```python
from build123d import *

# Parameters (mm, degrees)
F1_DEPTH = 3.81
F2_R     = 14.4183886526
F2_R_2   = 14.9688015553
F2_R_3   = 13.8673627738
F2_R_4   = 14.6123692091
F2_R_5   = 14.6887640566
F2_R_6   = 13.7656196585
F2_R_7   = 6.5271201163
F2_R_8   = 3.1776406916
F2_R_9   = 2.2295804693
F2_R_10  = 1.3934876863
F2_R_11  = 3.1159324266
F2_R_12  = 2.3730237654
F2_R_13  = 1.5391584656
F2_R_14  = 2.962596298
F2_R_15  = 2.2032977608
F2_R_16  = 2.9560338706
F2_R_17  = 2.3730243841
F2_R_18  = 1.4346833287
F2_R_19  = 1.5391578396
F2_R_20  = 2.8008757636
F2_R_21  = 2.094873282
F2_R_22  = 1.672185105
F2_R_23  = 3.2080502358
F2_R_24  = 2.1677587647
F2_R_25  = 1.3934881637
F3_DEPTH = 3.811
F4_SCALE = 0.6
F6_DEPTH = 2.287


with BuildPart() as f1:
    # F0 (on Top) → F1 (new body)
    with BuildSketch(Plane.XY):
        Polygon((21.5040096467, 37.2460372746), (-21.5040096467, 37.2460372746), (-43.0080192935, 0), (-21.5040096467, -37.2460372746), (21.5040096467, -37.2460372746), (43.0080192935, 0), align=None)
    extrude(amount=F1_DEPTH)

    # F2 (on face) → F3 (cut, through all)
    with BuildSketch(Plane.XY.offset(3.81)):
        with Locations((0, 37.2460372746)):
            Circle(F2_R)
        with Locations((-32.2560144701, 18.6230186373)):
            Circle(F2_R_2)
        with Locations((-32.2560144701, -18.6230186373)):
            Circle(F2_R_3)
        with Locations((0, -37.2460372746)):
            Circle(F2_R_4)
        with Locations((32.2560144701, -18.6230186373)):
            Circle(F2_R_5)
        with Locations((31.3001683758, 20.2785926369)):
            Circle(F2_R_6)
        Circle(F2_R_7)
        with Locations((-12.8094833344, 20.49517259)):
            Circle(F2_R_8)
        with Locations((-9.065172635, 13.0065521225)):
            Circle(F2_R_9)
        with Locations((-5.9120692313, 7.2915516794)):
            Circle(F2_R_10)
        with Locations((11.8241384625, 21.8746569008)):
            Circle(F2_R_11)
        with Locations((9.0651735663, 14.3860345706)):
            Circle(F2_R_12)
        with Locations((5.9120692313, 8.2768965513)):
            Circle(F2_R_13)
        with Locations((27.5896564126, 0)):
            Circle(F2_R_14)
        with Locations((18.9186222851, 0)):
            Circle(F2_R_15)
        with Locations((13.5977584869, -23.2541374862)):
            Circle(F2_R_16)
        with Locations((9.4593111426, -15.1743106544)):
            Circle(F2_R_17)
        with Locations((5.1237940788, -9.6563789994)):
            Circle(F2_R_18)
        with Locations((10.4446560144, 0)):
            Circle(F2_R_19)
        with Locations((-14.3860345706, -21.4805174619)):
            Circle(F2_R_20)
        with Locations((-10.4446560144, -14.7801730782)):
            Circle(F2_R_21)
        with Locations((-7.2915512137, -9.2622414231)):
            Circle(F2_R_22)
        with Locations((-26.2101721019, 0)):
            Circle(F2_R_23)
        with Locations((-17.9332755506, 0)):
            Circle(F2_R_24)
        with Locations((-11.2329311669, 0)):
            Circle(F2_R_25)
    extrude(amount=-F3_DEPTH, mode=Mode.SUBTRACT)


with BuildPart() as f1_1:
    # F4: moved
    add(f1.part.scale(F4_SCALE))

    # F5 (on face) → F6 (cut, through all)
    with BuildSketch(Plane.XY.offset(2.286)):
        Polygon((2.2348568425, 7.9494534601), (3.6136271371, 11.252985526), (0.8978448914, 13.585121549), (-2.1593711371, 11.7229288117), (-1.333052308, 8.2398943834), align=None)
        with BuildLine():
            ThreePointArc((-11.0931667862, 7.648402428), (-11.1968162546, 7.4148027366), (-11.3070701633, 7.1842466615))
            Line((-11.3070701633, 7.1842466615), (-11.2320397263, 3.9913941449))
            Line((-11.2320397263, 3.9913941449), (-7.8024840145, 2.9654900284))
            Line((-7.8024840145, 2.9654900284), (-5.7670002214, 5.9101695295))
            Line((-5.7670002214, 5.9101695295), (-7.9385577654, 8.7559856636))
            Line((-7.9385577654, 8.7559856636), (-11.0931667862, 7.648402428))
        make_face()
        Polygon((-6.4694317065, -5.274404355), (-8.0018570639, -2.0392839306), (-11.5521849025, -2.4969998625), (-12.2139828207, -6.0150042899), (-9.0726685891, -7.7315346668), align=None)
        Polygon((-2.2348568425, -7.9494534601), (-3.6136271371, -11.252985526), (-0.8978448914, -13.585121549), (2.1593711371, -11.7229288117), (1.333052308, -8.2398943834), align=None)
        with BuildLine():
            Line((5.7670002214, -5.9101695295), (7.9385577654, -8.7559856636))
            Line((7.9385577654, -8.7559856636), (11.3097934002, -7.5723448233))
            ThreePointArc((11.3097934002, -7.5723448233), (11.3128298264, -7.5655706667), (11.3158719575, -7.5587990702))
            Line((11.3158719575, -7.5587990702), (11.2320397263, -3.9913941449))
            Line((11.2320397263, -3.9913941449), (7.8024840145, -2.9654900284))
            Line((7.8024840145, -2.9654900284), (5.7670002214, -5.9101695295))
        make_face()
        Polygon((8.0018570639, 2.0392839306), (11.5521849025, 2.4969998625), (12.2139828207, 6.0150042899), (9.0726685891, 7.7315346668), (6.4694317065, 5.274404355), align=None)
    extrude(amount=-F6_DEPTH, mode=Mode.SUBTRACT)


solid = f1_1.part
```
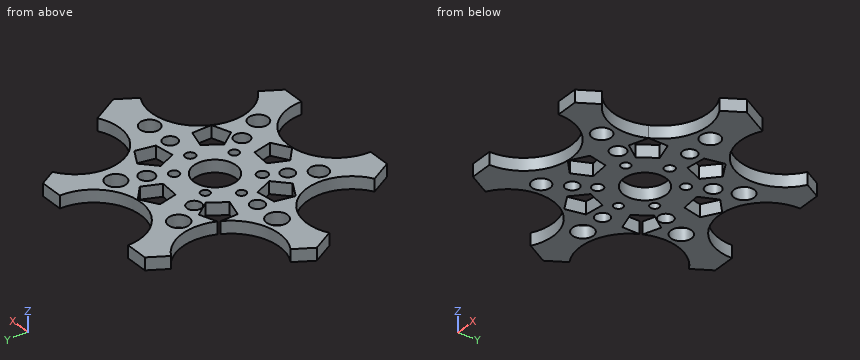
CAD build for the part. Positions are in the model's coordinates, mm. Round coordinates to 2 decimals unless told otherwise and drop trailing zeros. Order: outer loops, then holes, each group sorted by start corner. A loop starts at its lowest first (then second) coordinate and runs counter-clockwise, first axis right, second up. Notation, with made-up numbers: (-38, 67) -> (16, 67) arc R20 cw to (16, 92) -> close; hole circle Ø11 at (-39.5, 64). An arc over 180 degrees is marked (long way). One line per question, with ' | ' between items.
Q1. Slice it at C-C (z = 0.5). Give the number of separate pieces and of enclosed holes in the cut face, then the cut area to 3 significant figures.
Completed:
separate pieces: 1 | enclosed holes: 23 | area: 735 mm^2
Q2. Probe probe 1 along Y at (x, z) = (14, 0.25); probe 2 along X at (y, z) = (-7, 1.3); probe 3 along X at (y, z) = (-17, 1.65). List the from-to ranges inside material, lowest first.
Completed:
probe 1: y = -20.45 to -18.17, -4.17 to 5.43, 18.9 to 20.45 | probe 2: x = -12.16 to -10.41, -8.3 to 6.6, 11.3 to 11.59 | probe 3: x = -13.41 to -6.95, 6.95 to 12.74
Q3. Slice it at B-B (x = 0). Write the cut outline in (y, z).
Completed:
outline: (-13.58, 0) -> (-13.04, 0) -> (-13.04, 2.29) -> (-13.58, 2.29) -> close; (-8.13, 0) -> (-3.92, 0) -> (-3.92, 2.29) -> (-8.13, 2.29) -> close; (3.92, 0) -> (8.13, 0) -> (8.13, 2.29) -> (3.92, 2.29) -> close; (13.04, 0) -> (13.7, 0) -> (13.7, 2.29) -> (13.04, 2.29) -> close
Q4. Drop a flat-ended pin along its axis: pin 1 (1.5 mm diameter, centred on x = 3.07, y = -5.79, fed in from +Z). Give the stop position or say it passes through.
Completed:
pin 1: passes through
Q5. Slice it at A-A (y = 16.5). Write the cut outline in (x, z), then the cut area to 3 significant figures.
Completed:
outline: (-12.12, 0) -> (-6.38, 0) -> (-6.38, 2.29) -> (-12.12, 2.29) -> close; (6.38, 0) -> (11.75, 0) -> (11.75, 2.29) -> (6.38, 2.29) -> close | area: 25.4 mm^2
